Build history of the part. All positions in model axes, mm. Face numbers are marked on the shaded views. Give positions to 0.01 mm unless a question says otherwise; leave off trailing zeros. Write each loop counter-clockwise with the first axis right and the second up, starting at its lowest first coordinate (ties: lowest second). Pieces come first, ordered by that corner, then holes.
from build123d import *

# Parameters (mm, degrees)
F0_W     = 55
F0_H     = 42.3
F0_R     = 4.375
F0_R_2   = 7.825
F1_DEPTH = 15
F2_W     = 4.2
F2_H     = 4
F3_DEPTH = 3.5
F4_R     = 0.75


with BuildPart() as f1:
    # F0 (on Front) → F1 (new body)
    with BuildSketch(Plane.XZ):
        Rectangle(F0_W, F0_H)
        with Locations((-17.5, 0)):
            Circle(F0_R, mode=Mode.SUBTRACT)
        Circle(F0_R_2, mode=Mode.SUBTRACT)
        with Locations((17.5, 0)):
            Circle(F0_R, mode=Mode.SUBTRACT)
    extrude(amount=F1_DEPTH)

    # F2 (on face) → F3 (join)
    with BuildSketch(Plane(origin=(0, 0, 0), x_dir=(-1, 0, 0), z_dir=(0, 1, 0))):
        with Locations((0, 19.15)):
            Rectangle(F2_W, F2_H)
        with Locations((0, -19.15)):
            Rectangle(F2_W, F2_H)
        Polygon((-17.5, 17.15), (-17.5, 21.15), (-27.5, 21.15), (-27.5, 11.15), (-23.5, 11.15), (-23.5, 17.15), align=None)
        Polygon((-23.5, -11.15), (-27.5, -11.15), (-27.5, -21.15), (-17.5, -21.15), (-17.5, -17.15), (-23.5, -17.15), align=None)
        Polygon((27.5, 21.15), (17.5, 21.15), (17.5, 17.15), (23.5, 17.15), (23.5, 11.15), (27.5, 11.15), align=None)
        Polygon((27.5, -21.15), (27.5, -11.15), (23.5, -11.15), (23.5, -17.15), (17.5, -17.15), (17.5, -21.15), align=None)
    extrude(amount=F3_DEPTH)

    # F4
    f4_edges = [f1.edges().sort_by_distance(p)[0] for p in [
        (0, 3.5, -17.15),
        (0, 3.5, 17.15),
        (20.5, 3.5, 17.15),
        (23.5, 3.5, 14.15),
        (23.5, 3.5, -14.15),
        (20.5, 3.5, -17.15),
        (-20.5, 3.5, -17.15),
        (-23.5, 3.5, -14.15),
        (-23.5, 3.5, 14.15),
        (-20.5, 3.5, 17.15),
    ]]
    fillet(f4_edges, radius=F4_R)


solid = f1.part
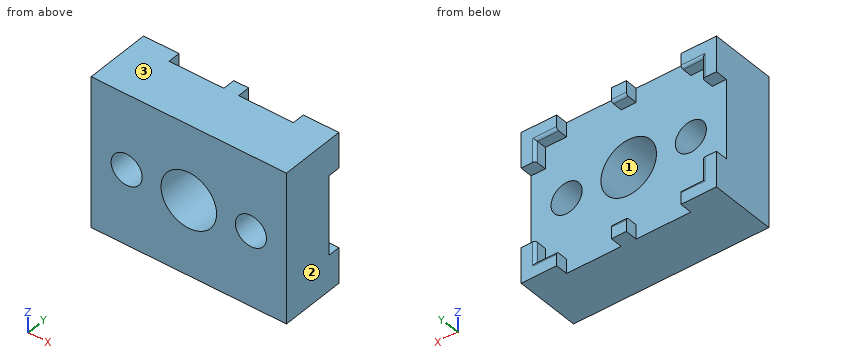
1. Saw through at A-A on x = 0. Give the cut face in (y, z) (3 decimals), plus the area to 3 significant figures.
2. Saw through at B-B on y = -0.75. Give the cut face in (x, z) (3 decimals), plus the area to 3 significant figures.
3. Saw through at D-D on z = 15.5. Give the cut face in (x, y), plus the area to 3 significant figures.
4. Mould opens along Z. For the marked faces 1, 2 and 3 say: pulls with the +Z half, pulls with the -Z half, needs draft (parallel to the pull), parting line crosses it, or undercut.
5. Drop a flat-ended pin along its axis: pin 1 (4 mm diameter, centred on x = -6, z = -2.5, fed in from +Y). Give the stop position or say it passes through.
6. Saw through at C-C on z = 0. Give the cut face in (x, y) (3 decimals).
7. Drill centre lines: line 1 along Z through (x, y) = (-17.5, -3.75) (3 decimals); line 2 along Z through (x, y) = (0, -5.25) (3 decimals); line 3 along Y through (x, z) = (3.5, 14.5). Where is each one in solid material? Low to high.
Outcome:
1. outline: (-15, -21.15) - (3.5, -21.15) - (3.5, -17.9) arc R0.75 ccw to (2.75, -17.15) - (0, -17.15) - (0, -7.825) - (-15, -7.825) - close; (-15, 7.825) - (0, 7.825) - (0, 17.15) - (2.75, 17.15) arc R0.75 ccw to (3.5, 17.9) - (3.5, 21.15) - (-15, 21.15) - close
1. area: 428 mm2
2. outline: (-27.5, -21.15) - (27.5, -21.15) - (27.5, 21.15) - (-27.5, 21.15) - close; hole circle Ø8.75 at (-17.5, 0); hole circle Ø15.65 at (0, 0); hole circle Ø8.75 at (17.5, 0)
2. area: 2,010 mm2
3. outline: (-27.5, -15) - (27.5, -15) - (27.5, 3.5) - (24.25, 3.5) arc R0.75 ccw to (23.5, 2.75) - (23.5, 0) - (-23.5, 0) - (-23.5, 2.75) arc R0.75 ccw to (-24.25, 3.5) - (-27.5, 3.5) - close
3. area: 853 mm2
4. face 1: undercut
4. face 2: needs draft
4. face 3: pulls with the +Z half
5. pin 1: stops at y = 0
6. outline: (-27.5, -15) - (-21.875, -15) - (-21.875, 0) - (-27.5, 0) - close; (-13.125, -15) - (-7.825, -15) - (-7.825, 0) - (-13.125, 0) - close; (7.825, -15) - (13.125, -15) - (13.125, 0) - (7.825, 0) - close; (21.875, -15) - (27.5, -15) - (27.5, 0) - (21.875, 0) - close
7. line 1: z = -21.15 to -4.375, 4.375 to 21.15
7. line 2: z = -21.15 to -7.825, 7.825 to 21.15
7. line 3: y = -15 to 0
